Design review of the part built by this model. Coordinates are the model's own, in mm. Round coordinates to 2 decimals unless told otherwise and drop trailing zeros. Loops run counter-clockwise (first coordinate to the right, second up) from the corner with the lowest first, then second, coordinate; pieces in that order, holes last. Notation, with made-up numbers: (15.25, -6) - (64.25, -6) arc R14 cw to (64.25, 20) - close; hole circle Ø1 at (-26, 17.25). An arc over 180 degrees is marked (long way). Return JSON: item names as keys, results as strings. Group by question number.
(1) We need section A-A, the plane x = 18. Write out the cut boundary in (y, z), and give its area (3 significant figures).
(2) We need section D-D, the plane x = 77. Write out the cut boundary in (y, z), and give its area (3 significant figures).
(3) We need section C-C, the plane y = -20.5. Write out the cut boundary in (x, z) (3 decimals), and give its area (3 significant figures).
(4) We need section B-B, the plane z = 0.7. Write out the cut boundary in (x, y).
(5) Wall thickness on L1, parallel to X at y = 12, z = 1.5; L2, parallel to X at y = -37, z = 2.5; L3, parallel to X at y = -34.5, z = 2.4 (3 decimals): over which ranges is each line inside the solid? List them lowest first. Write a range as [from, to].
(6) Clearance check with flat-ended pins moving along their axes: pin 1 (1 mm diameter, centred on x = -4, z = 0.5, fed in from +Y); pin 2 (1.5 mm diameter, centred on x = -13, z = 2, fed in from -Y); pin 3 (0.9 mm diameter, centred on y = 12, z = 1.5, fed in from +X). State where each tip first meets the part, or that it passes through.
Autodesk Inventor part; units mm, degrees
ref_plane "YZ Plane" through (0, 0, 0) normal (1, 0, 0) x (0, 1, 0)
ref_plane "XZ Plane" through (0, 0, 0) normal (0, 1, 0) x (-1, 0, 0)
ref_plane "XY Plane" through (0, 0, 0) normal (0, 0, 1) x (1, 0, 0)
sketch "Sketch1" plane through (0, 0, 0) normal (0, 0, 1) x (1, 0, 0)
  line L0 (0, 19.5) -> (50, 19.5)
  line L1 (50, 19.5) -> (50, 6.5)
  line L2 (50, 6.5) -> (0, 6.5)
  line L3 (0, 6.5) -> (0, 19.5)
  line L4 (50, 19.5) -> (65, 19.5)
  line L5 (65, 19.5) -> (65, 0)
  line L6 (65, 0) -> (50, 0)
  line L7 (50, 0) -> (50, 19.5)
  line L8 (65, 0) -> (0, 0)
  line L9 (0, 0) -> (0, -16)
  line L10 (0, -16) -> (65, -16)
  line L11 (65, -16) -> (65, 0)
  line L12 (0, 0) -> (-68.75, -55)
  line L13 (-68.75, -55) -> (-48.75, -55)
  line L14 (-48.75, -55) -> (0, -16)
  line L15 (65, -16) -> (113.75, -55)
  line L16 (113.75, -55) -> (133.75, -55)
  line L17 (133.75, -55) -> (65, 0)
  point P0 (50, 6.5)
  point P1 (50, 0)
  dimension "d0" = 6.5
  dimension "d1" = 13
  dimension "d2" = 50
  dimension "d3" = 15
  dimension "d4" = 16
  dimension "d5" = 20
  dimension "d6" = 20
  dimension "d7" = 55
extrude "Extrusion1" add sketch "Sketch1" along normal blind 3
properties part number "Support_base"
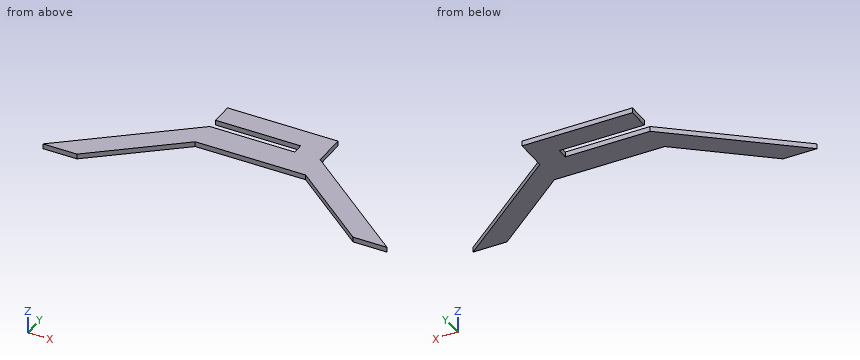
Solutions:
{
 "1": {"outline": "(-16, 0) - (0, 0) - (0, 3) - (-16, 3) - close; (6.5, 0) - (19.5, 0) - (19.5, 3) - (6.5, 3) - close", "area": "87.0 mm^2"},
 "2": {"outline": "(-25.6, 0) - (-9.6, 0) - (-9.6, 3) - (-25.6, 3) - close", "area": "48.0 mm^2"},
 "3": {"outline": "(-25.625, 0) - (-5.625, 0) - (-5.625, 3) - (-25.625, 3) - close; (70.625, 0) - (90.625, 0) - (90.625, 3) - (70.625, 3) - close", "area": "120 mm^2"},
 "4": {"outline": "(-68.75, -55) - (-48.75, -55) - (0, -16) - (65, -16) - (113.75, -55) - (133.75, -55) - (65, 0) - (65, 19.5) - (0, 19.5) - (0, 6.5) - (50, 6.5) - (50, 0) - (0, 0) - close"},
 "5": {"L1": "[0, 65]", "L2": "[-46.25, -26.25], [91.25, 111.25]", "L3": "[-43.125, -23.125], [88.125, 108.125]"},
 "6": {"pin 1": "y = -2.8", "pin 2": "y = -27", "pin 3": "x = 65"}
}
